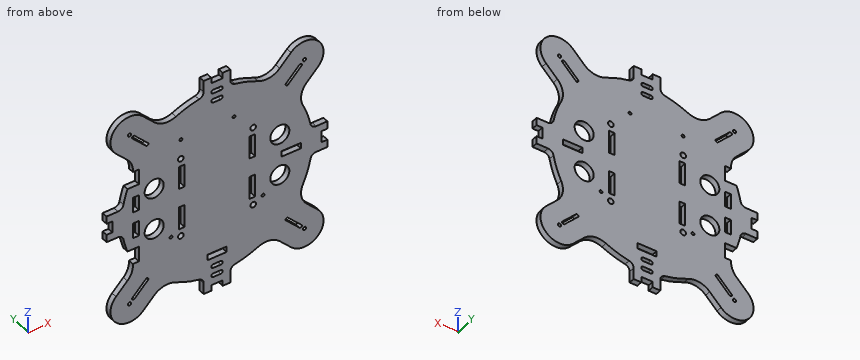
from build123d import *

# Parameters (mm, degrees)
ESQUISSE1_R             = 0.85
ESQUISSE1_R_2           = 1.5
ESQUISSE1_R_3           = 0.75
ESQUISSE1_R_4           = 5
ESQUISSE1_W             = 3
ESQUISSE1_H             = 12
ESQUISSE1_W_2           = 10
ESQUISSE1_H_2           = 3
BOSS_EXTRU_1_DEPTH      = 3
CONG_1_R                = 10
CONG_2_R                = 3
ENL_V_MAT_EXTRU_1_REACH = 84.079
ESQUISSE4_W             = 10
ESQUISSE4_H             = 8
ESQUISSE4_W_2           = 3


with BuildPart() as part:
    # Esquisse1 → Boss.-Extru.1 (new body)
    with BuildSketch(Plane(origin=(0, 0, 0), x_dir=(1, 0, 0), z_dir=(0, 1, 0))):
        with BuildLine():
            Line((-38.890872965, -53.033008589), (-27.56994834, -41.712083963))
            ThreePointArc((-27.56994834, -41.712083963), (-17.718994127, -46.755077234), (-7, -49.507575178))
            Line((-7, -49.507575178), (-7, -58))
            Line((-7, -58), (-3, -58))
            Line((-3, -58), (-3, -55))
            Line((-3, -55), (3, -55))
            Line((3, -55), (3, -58))
            Line((3, -58), (7, -58))
            Line((7, -58), (7, -49.507575178))
            ThreePointArc((7, -49.507575178), (17.718994127, -46.755077234), (27.56994834, -41.712083963))
            Line((27.56994834, -41.712083963), (38.890872965, -53.033008589))
            ThreePointArc((38.890872965, -53.033008589), (53.033008589, -53.033008589), (53.033008589, -38.890872965))
            Line((53.033008589, -38.890872965), (41.712083963, -27.56994834))
            ThreePointArc((41.712083963, -27.56994834), (46.755077234, -17.718994127), (49.507575178, -7))
            Line((49.507575178, -7), (58, -7))
            Line((58, -7), (58, -3))
            Line((58, -3), (55, -3))
            Line((55, -3), (55, 3))
            Line((55, 3), (58, 3))
            Line((58, 3), (58, 7))
            Line((58, 7), (49.507575178, 7))
            ThreePointArc((49.507575178, 7), (46.755077234, 17.718994127), (41.712083963, 27.56994834))
            Line((41.712083963, 27.56994834), (53.033008589, 38.890872965))
            ThreePointArc((53.033008589, 38.890872965), (53.033008589, 53.033008589), (38.890872965, 53.033008589))
            Line((38.890872965, 53.033008589), (27.56994834, 41.712083963))
            ThreePointArc((27.56994834, 41.712083963), (17.718994127, 46.755077234), (7, 49.507575178))
            Line((7, 49.507575178), (7, 58))
            Line((7, 58), (3, 58))
            Line((3, 58), (3, 55))
            Line((3, 55), (-3, 55))
            Line((-3, 55), (-3, 58))
            Line((-3, 58), (-7, 58))
            Line((-7, 58), (-7, 49.507575178))
            ThreePointArc((-7, 49.507575178), (-17.718994127, 46.755077234), (-27.56994834, 41.712083963))
            Line((-27.56994834, 41.712083963), (-38.890872965, 53.033008589))
            ThreePointArc((-38.890872965, 53.033008589), (-53.033008589, 53.033008589), (-53.033008589, 38.890872965))
            Line((-53.033008589, 38.890872965), (-41.712083963, 27.56994834))
            ThreePointArc((-41.712083963, 27.56994834), (-46.755077234, 17.718994127), (-49.507575178, 7))
            Line((-49.507575178, 7), (-58, 7))
            Line((-58, 7), (-58, 3))
            Line((-58, 3), (-55, 3))
            Line((-55, 3), (-55, -3))
            Line((-55, -3), (-58, -3))
            Line((-58, -3), (-58, -7))
            Line((-58, -7), (-49.507575178, -7))
            ThreePointArc((-49.507575178, -7), (-46.755077234, -17.718994127), (-41.712083963, -27.56994834))
            Line((-41.712083963, -27.56994834), (-53.033008589, -38.890872965))
            ThreePointArc((-53.033008589, -38.890872965), (-53.033008589, -53.033008589), (-38.890872965, -53.033008589))
        make_face()
        with Locations(Location((-45.961940777, -45.961940777, 0), (0, 0, 270))):
            Circle(ESQUISSE1_R, mode=Mode.SUBTRACT)
        with Locations(Location((-45.961940777, 45.961940777, 0), (0, 0, 270))):
            Circle(ESQUISSE1_R, mode=Mode.SUBTRACT)
        with Locations(Location((45.961940777, 45.961940777, 0), (0, 0, 270))):
            Circle(ESQUISSE1_R, mode=Mode.SUBTRACT)
        with Locations(Location((45.961940777, -45.961940777, 0), (0, 0, 270))):
            Circle(ESQUISSE1_R, mode=Mode.SUBTRACT)
        with Locations(Location((-19, 21, 0), (0, 0, 270))):
            Circle(ESQUISSE1_R_2, mode=Mode.SUBTRACT)
        with Locations(Location((19, 21, 0), (0, 0, 270))):
            Circle(ESQUISSE1_R_2, mode=Mode.SUBTRACT)
        with Locations(Location((19, -21, 0), (0, 0, 270))):
            Circle(ESQUISSE1_R_2, mode=Mode.SUBTRACT)
        with Locations(Location((-19, -21, 0), (0, 0, 270))):
            Circle(ESQUISSE1_R_2, mode=Mode.SUBTRACT)
        with Locations(Location((24.15, 18.1, 0), (0, 0, 270))):
            Circle(ESQUISSE1_R_3, mode=Mode.SUBTRACT)
        with Locations(Location((-24.15, 19.4, 0), (0, 0, 270))):
            Circle(ESQUISSE1_R_3, mode=Mode.SUBTRACT)
        with Locations(Location((-18.95, -31.4, 0), (0, 0, 270))):
            Circle(ESQUISSE1_R_3, mode=Mode.SUBTRACT)
        with Locations(Location((8.95, -31.4, 0), (0, 0, 270))):
            Circle(ESQUISSE1_R_3, mode=Mode.SUBTRACT)
        with Locations(Location((-33, 11, 0), (0, 0, 270))):
            Circle(ESQUISSE1_R_4, mode=Mode.SUBTRACT)
        with Locations(Location((33, 11, 0), (0, 0, 270))):
            Circle(ESQUISSE1_R_4, mode=Mode.SUBTRACT)
        with Locations(Location((33, -11, 0), (0, 0, 270))):
            Circle(ESQUISSE1_R_4, mode=Mode.SUBTRACT)
        with Locations(Location((-33, -11, 0), (0, 0, 270))):
            Circle(ESQUISSE1_R_4, mode=Mode.SUBTRACT)
        with Locations((-18.5, 11)):
            Rectangle(ESQUISSE1_W, ESQUISSE1_H, mode=Mode.SUBTRACT)
        with Locations((18.5, 11)):
            Rectangle(ESQUISSE1_W, ESQUISSE1_H, mode=Mode.SUBTRACT)
        with Locations((18.5, -11)):
            Rectangle(ESQUISSE1_W, ESQUISSE1_H, mode=Mode.SUBTRACT)
        with Locations((-18.5, -11)):
            Rectangle(ESQUISSE1_W, ESQUISSE1_H, mode=Mode.SUBTRACT)
        with BuildLine():
            Line((-44.370950519, -43.310290348), (-37.299882708, -36.239222536))
            ThreePointArc((-37.299882708, -36.239222536), (-36.239222536, -36.239222536), (-36.239222536, -37.299882708))
            Line((-36.239222536, -37.299882708), (-43.310290348, -44.370950519))
            ThreePointArc((-43.310290348, -44.370950519), (-44.370950519, -44.370950519), (-44.370950519, -43.310290348))
        make_face(mode=Mode.SUBTRACT)
        with BuildLine():
            Line((-43.310290348, 44.370950519), (-36.239222536, 37.299882708))
            ThreePointArc((-36.239222536, 37.299882708), (-36.239222536, 36.239222536), (-37.299882708, 36.239222536))
            Line((-37.299882708, 36.239222536), (-44.370950519, 43.310290348))
            ThreePointArc((-44.370950519, 43.310290348), (-44.370950519, 44.370950519), (-43.310290348, 44.370950519))
        make_face(mode=Mode.SUBTRACT)
        with BuildLine():
            Line((44.370950519, 43.310290348), (37.299882708, 36.239222536))
            ThreePointArc((37.299882708, 36.239222536), (36.239222536, 36.239222536), (36.239222536, 37.299882708))
            Line((36.239222536, 37.299882708), (43.310290348, 44.370950519))
            ThreePointArc((43.310290348, 44.370950519), (44.370950519, 44.370950519), (44.370950519, 43.310290348))
        make_face(mode=Mode.SUBTRACT)
        with BuildLine():
            Line((43.310290348, -44.370950519), (36.239222536, -37.299882708))
            ThreePointArc((36.239222536, -37.299882708), (36.239222536, -36.239222536), (37.299882708, -36.239222536))
            Line((37.299882708, -36.239222536), (44.370950519, -43.310290348))
            ThreePointArc((44.370950519, -43.310290348), (44.370950519, -44.370950519), (43.310290348, -44.370950519))
        make_face(mode=Mode.SUBTRACT)
        with BuildLine():
            Line((-2, -44), (2, -44))
            ThreePointArc((2, -44), (3, -45), (2, -46))
            Line((2, -46), (-2, -46))
            ThreePointArc((-2, -46), (-3, -45), (-2, -44))
        make_face(mode=Mode.SUBTRACT)
        with BuildLine():
            Line((-2, -49), (2, -49))
            ThreePointArc((2, -49), (3, -50), (2, -51))
            Line((2, -51), (-2, -51))
            ThreePointArc((-2, -51), (-3, -50), (-2, -49))
        make_face(mode=Mode.SUBTRACT)
        with BuildLine():
            Line((-2, 49), (2, 49))
            ThreePointArc((2, 49), (3, 50), (2, 51))
            Line((2, 51), (-2, 51))
            ThreePointArc((-2, 51), (-3, 50), (-2, 49))
        make_face(mode=Mode.SUBTRACT)
        with BuildLine():
            Line((-2, 44), (2, 44))
            ThreePointArc((2, 44), (3, 45), (2, 46))
            Line((2, 46), (-2, 46))
            ThreePointArc((-2, 46), (-3, 45), (-2, 44))
        make_face(mode=Mode.SUBTRACT)
        with Locations((39, 0)):
            Rectangle(ESQUISSE1_W_2, ESQUISSE1_H_2, mode=Mode.SUBTRACT)
        with Locations((0, 39)):
            Rectangle(ESQUISSE1_W_2, ESQUISSE1_H_2, mode=Mode.SUBTRACT)
    extrude(amount=BOSS_EXTRU_1_DEPTH)

    # Congé1
    cong_1_edges = [part.edges().sort_by_distance(p)[0] for p in [
        (-27.56994834, 1.5, 41.712083963),
        (-41.712083963, 1.5, 27.56994834),
        (-41.712083963, 1.5, -27.56994834),
        (-27.56994834, 1.5, -41.712083963),
        (27.56994834, 1.5, -41.712083963),
        (41.712083963, 1.5, -27.56994834),
        (41.712083963, 1.5, 27.56994834),
        (27.56994834, 1.5, 41.712083963),
    ]]
    fillet(cong_1_edges, radius=CONG_1_R)

    # Congé2
    cong_2_edges = [part.edges().sort_by_distance(p)[0] for p in [
        (7, 1.5, 49.507575178),
        (-7, 1.5, 49.507575178),
        (-49.507575178, 1.5, 7),
        (-49.507575178, 1.5, -7),
        (-7, 1.5, -49.507575178),
        (7, 1.5, -49.507575178),
        (49.507575178, 1.5, -7),
        (49.507575178, 1.5, 7),
    ]]
    fillet(cong_2_edges, radius=CONG_2_R)

    # Esquisse4 → Enlèv. mat.-Extru.1 (cut, up to next)
    with BuildSketch(Plane(origin=(0, 3, 0), x_dir=(1, 0, 0), z_dir=(0, 1, 0)), mode=Mode.PRIVATE) as enl_v_mat_extru_1_sk1:
        with Locations((-46, 21)):
            Rectangle(ESQUISSE4_W, ESQUISSE4_H)
    enl_v_mat_extru_1_tool1 = extrude(enl_v_mat_extru_1_sk1.sketch, amount=-ENL_V_MAT_EXTRU_1_REACH, mode=Mode.PRIVATE) & part.part
    # Esquisse4 → Enlèv. mat.-Extru.1 (cut, up to next)
    with BuildSketch(Plane(origin=(0, 3, 0), x_dir=(1, 0, 0), z_dir=(0, 1, 0)), mode=Mode.PRIVATE) as enl_v_mat_extru_1_sk2:
        with Locations((-42.5, 7)):
            Rectangle(ESQUISSE4_W_2, ESQUISSE4_H)
    enl_v_mat_extru_1_tool2 = extrude(enl_v_mat_extru_1_sk2.sketch, amount=-ENL_V_MAT_EXTRU_1_REACH, mode=Mode.PRIVATE) & part.part
    # Esquisse4 → Enlèv. mat.-Extru.1 (cut, up to next)
    with BuildSketch(Plane(origin=(0, 3, 0), x_dir=(1, 0, 0), z_dir=(0, 1, 0)), mode=Mode.PRIVATE) as enl_v_mat_extru_1_sk3:
        with Locations((-46, -21)):
            Rectangle(ESQUISSE4_W, ESQUISSE4_H)
    enl_v_mat_extru_1_tool3 = extrude(enl_v_mat_extru_1_sk3.sketch, amount=-ENL_V_MAT_EXTRU_1_REACH, mode=Mode.PRIVATE) & part.part
    # Esquisse4 → Enlèv. mat.-Extru.1 (cut, up to next)
    with BuildSketch(Plane(origin=(0, 3, 0), x_dir=(1, 0, 0), z_dir=(0, 1, 0)), mode=Mode.PRIVATE) as enl_v_mat_extru_1_sk4:
        with Locations((-42.5, -7)):
            Rectangle(ESQUISSE4_W_2, ESQUISSE4_H)
    enl_v_mat_extru_1_tool4 = extrude(enl_v_mat_extru_1_sk4.sketch, amount=-ENL_V_MAT_EXTRU_1_REACH, mode=Mode.PRIVATE) & part.part
    add(enl_v_mat_extru_1_tool1.solids().sort_by_distance((-46, 3, -21))[0], mode=Mode.SUBTRACT)
    add(enl_v_mat_extru_1_tool2.solids().sort_by_distance((-42.5, 3, -7))[0], mode=Mode.SUBTRACT)
    add(enl_v_mat_extru_1_tool3.solids().sort_by_distance((-46, 3, 21))[0], mode=Mode.SUBTRACT)
    add(enl_v_mat_extru_1_tool4.solids().sort_by_distance((-42.5, 3, 7))[0], mode=Mode.SUBTRACT)


solid = part.part
CAD build for the part. Positions are in the model's coordinates, mm. Coordinates: 2 decimals unless noted, no trailing zeros. Write each loop counter-clockwise with the first axis right and the second up, starting at its lowest first coordinate (ties: lowest second). Pieces come first, ordered by that corner, then holes. Notation, with made-up numbers: (76, -33) - (92, -33) arc R25 cw to (92, 0) - close; hole circle Ø5 at (35, 50.5). An arc over 180 degrees is marked (long way). Use a Markdown table: item, result. Add a question column.
Item 1: Drill centre lines: L1, parallel to Z at x = -2, y = 0.3; L2, parallel to Z at x = -40, y = 1.35; L3, parallel to X at y = 2.85, z = -12.5. Where is each one in solid material? Low to high. Write a range as from..to.
Item 2: Band-saw the part on D-D, the plane x = -11. Give the cut face in (y, z) (3 decimals), and give its area (3 significant figures).
Item 3: Band-saw the part on A-A, the plane x = 40.5. Give the cut face in (y, z).
Item 4: Flat gauge pins, fed straight in: pin 1 (1 mm diameter, centred on y = 2.5, z = 8.5, fed in from +X); pin 2 (1.5 mm diameter, centred on x = -42, y = 2, fed in from +Z); pin 3 (1.5 mm diameter, centred on x = 0, y = 1.5, fed in from -Z); pin 4 (1.4 mm diameter, centred on x = -45.96, z = 45.96, fed in from -Y). Where does each tip first touch, or does it go through?
Item 5: Band-saw the part on B-B, the plane x = -34.5. Give the cut face in (y, z).
Item 6: Band-saw the part on C-C, the plane y = 2.55. Give the number of separate pieces and of enclosed holes in the cut face, and give its area (3 significant figures).
Numbers:
| question | item | result |
|---|---|---|
| 1 | L1 | -55..-51, -49..-46, -44..-40.5, -37.5..44, 46..49, 51..55 |
| 1 | L2 | -53.99..-41.06, -38.94..38.94, 41.06..53.99 |
| 1 | L3 | -48.41..-37.77, -28.23..-20, -17..17, 20..28.23, 37.77..48.41 |
| 2 | outline | (0, -48.775) - (3, -48.775) - (3, 48.775) - (0, 48.775) - close |
| 2 | area | 293 mm2 |
| 3 | outline | (0, -54.34) - (3, -54.34) - (3, -41.56) - (0, -41.56) - close; (0, -39.44) - (3, -39.44) - (3, -1.5) - (0, -1.5) - close; (0, 1.5) - (3, 1.5) - (3, 39.44) - (0, 39.44) - close; (0, 41.56) - (3, 41.56) - (3, 54.34) - (0, 54.34) - close |
| 4 | pin 1 | x = 49.81 |
| 4 | pin 2 | z = 55.43 |
| 4 | pin 3 | z = -55 |
| 4 | pin 4 | through |
| 5 | outline | (0, -48.64) - (3, -48.64) - (3, -15.77) - (0, -15.77) - close; (0, -6.23) - (3, -6.23) - (3, 6.23) - (0, 6.23) - close; (0, 15.77) - (3, 15.77) - (3, 48.64) - (0, 48.64) - close |
| 6 | separate pieces | 1 |
| 6 | enclosed holes | 32 |
| 6 | area | 9,390 mm2 |
